from build123d import *

# Parameters (mm, degrees)
SKETCH2_W           = 42
SKETCH2_H           = 8.4
BOSS_EXTRUDE1_DEPTH = 2
SKETCH3_W           = 3.55
SKETCH3_H           = 8.4
SKETCH3_W_2         = 10
BOSS_EXTRUDE2_DEPTH = 2
FILLET1_R           = 2
SKETCH4_R           = 1
CUT_EXTRUDE1_DEPTH  = 2
SKETCH5_W           = 20
SKETCH5_H           = 28
BOSS_EXTRUDE3_DEPTH = 7.5
FILLET2_R           = 2
SKETCH6_W           = 3.5
SKETCH6_H           = 22
CUT_EXTRUDE2_DEPTH  = 20
SKETCH7_W           = 44.314231138
SKETCH7_H           = 10.974489351
CUT_EXTRUDE3_DEPTH  = 4
SKETCH8_W           = 14
SKETCH8_H           = 4
CUT_EXTRUDE4_DEPTH  = 10


with BuildPart() as part:
    # Sketch2 → Boss-Extrude1 (new body)
    with BuildSketch(Plane.XY.offset(-7.754792002)):
        Rectangle(SKETCH2_W, SKETCH2_H)
    extrude(amount=BOSS_EXTRUDE1_DEPTH)

    # Sketch3 → Boss-Extrude2 (add)
    with BuildSketch(Plane.XY.offset(-5.754792002)):
        with Locations((-8.975, 0)):
            Rectangle(SKETCH3_W, SKETCH3_H)
        with Locations((8.975, 0)):
            Rectangle(SKETCH3_W, SKETCH3_H)
        Rectangle(SKETCH3_W_2, SKETCH3_H)
    extrude(amount=BOSS_EXTRUDE2_DEPTH)

    # Fillet1
    fillet1_edges = [part.edges().sort_by_distance(p)[0] for p in [
        (-21, 4.2, -6.754792002),
        (21, 4.2, -6.754792002),
        (21, -4.2, -6.754792002),
        (-21, -4.2, -6.754792002),
    ]]
    fillet(fillet1_edges, radius=FILLET1_R)

    # Sketch4 → Cut-Extrude1 (cut)
    with BuildSketch(Plane.XY.offset(-5.754792002)):
        with Locations((-17.75, 0)):
            Circle(SKETCH4_R)
        with Locations((17.75, 0)):
            Circle(SKETCH4_R)
    extrude(amount=-CUT_EXTRUDE1_DEPTH, mode=Mode.SUBTRACT)

    # Sketch5 → Boss-Extrude3 (add)
    with BuildSketch(Plane(origin=(0, 0, -7.754792002), x_dir=(-1, 0, 0), z_dir=(0, 0, -1))):
        Rectangle(SKETCH5_W, SKETCH5_H)
    extrude(amount=BOSS_EXTRUDE3_DEPTH)

    # Fillet2
    fillet2_edges = [part.edges().sort_by_distance(p)[0] for p in [
        (0, 14, -7.754792002),
        (0, -14, -7.754792002),
        (0, 14, -15.254792002),
        (0, -14, -15.254792002),
    ]]
    fillet(fillet2_edges, radius=FILLET2_R)

    # Sketch6 → Cut-Extrude2 (cut)
    with BuildSketch(Plane.ZY.offset(10)):
        with Locations((-11.504792002, 0)):
            Rectangle(SKETCH6_W, SKETCH6_H)
    extrude(amount=-CUT_EXTRUDE2_DEPTH, mode=Mode.SUBTRACT)

    # Sketch7 → Cut-Extrude3 (cut)
    with BuildSketch(Plane.XY.offset(-3.754792002)):
        with Locations((-0.219821089, -0.04579799)):
            Rectangle(SKETCH7_W, SKETCH7_H)
    extrude(amount=-CUT_EXTRUDE3_DEPTH, mode=Mode.SUBTRACT)

    # Sketch8 → Cut-Extrude4 (cut)
    with BuildSketch(Plane.XY.offset(-7.754792002)):
        with Locations((0, -12)):
            Rectangle(SKETCH8_W, SKETCH8_H)
    extrude(amount=-CUT_EXTRUDE4_DEPTH, mode=Mode.SUBTRACT)


solid = part.part
Here's how the part is built. I have some questions about the finished solid (model axes, mm). A direction names the side the tool comes from. Give positions to 0.01 mm unless a question says otherwise; leave off trailing zeros. Write each loop counter-clockwise with the first axis right and the second up, starting at its lowest first coordinate (ties: lowest second). Pieces come first, ordered by that corner, then holes. Notation, with made-up numbers: (78.25, 50) -> (86.25, 50) arc R34 cw to (86.25, 85) -> close; hole circle Ø2 at (-33.5, 61.5). An arc over 180 degrees is marked (long way). Use one line per item in the form item = value. Start each with the question number.
1. Thinking about a two-plate mould opening in X: for faces 1 (the face through (10, 0, -9)), 2 (the face through (7, -12, -11)), 3 (the face through (0, 0, -9.755)), 4 (the face through (-7, -12, -11)), which applies, +X half, -X half, draft (parallel to the pull), parting line (faces both ways), or undercut?
2. Imagine slicing it at D-D on x = 9.25. List the corners of the cut face in (y, z) for me, plus the area to 3 significant figures.
3. Imagine slicing it at C-C on x = -2.5. List the corners of the cut face in (y, z) for me.
4. Imagine slicing it at B-B on y = -8.5. List the corners of the cut face in (x, z) for me.
5. Imagine slicing it at A-A on z = -12.5. List the corners of the cut face in (x, y) for me, plus the area to 3 significant figures.
6. If I drill on L1, parallel to Z at x = -2, y = 6.25; L2, parallel to Y at x = 8.75, z = -12.75; L3, parallel to X at y = -12.5, z = -12.75, over which ranges is the centre line in solid material (lowest first)?
7. On a 3-axis mill with a long thin cutter (end or side, diameter ignored), from which of +Z, -Z, +X, -X, +Y, -Y can I reach the whole of each face in a straight line? I mean faces 5 (the face through (9, -14, -11)), 6 (the face through (8, -11, -12)). Say none if no direction works.
8. Will these pins go through, and if not, where does the flat tip stop? pin 1 Ø8 at (x, y) = (-6.5, -11) entering from +Z; pin 2 Ø1 at (x, z) = (2, -14.5) entering from -Y.
Entries:
q1.face_1 = +X half
q1.face_2 = undercut
q1.face_3 = draft
q1.face_4 = undercut
q2.outline = (-14, -13.25) arc R2 ccw to (-12, -15.25) -> (12, -15.25) arc R2 ccw to (14, -13.25) -> (14, -9.75) arc R2 ccw to (12, -7.75) -> (-12, -7.75) arc R2 ccw to (-14, -9.75) -> close; hole (-11, -13.25) -> (11, -13.25) -> (11, -9.75) -> (-11, -9.75) -> close
q2.area = 130 mm²
q3.outline = (-10, -15.25) -> (12, -15.25) arc R2 ccw to (14, -13.25) -> (14, -9.75) arc R2 ccw to (12, -7.75) -> (-10, -7.75) -> (-10, -9.75) -> (11, -9.75) -> (11, -13.25) -> (-10, -13.25) -> close
q4.outline = (-10, -15.25) -> (10, -15.25) -> (10, -13.25) -> (-10, -13.25) -> close; (-10, -9.75) -> (10, -9.75) -> (10, -7.75) -> (-10, -7.75) -> close
q5.outline = (-10, -14) -> (-7, -14) -> (-7, -11) -> (-10, -11) -> close; (-10, 11) -> (10, 11) -> (10, 14) -> (-10, 14) -> close; (7, -14) -> (10, -14) -> (10, -11) -> (7, -11) -> close
q5.area = 78.0 mm²
q6.L1 = -15.25 to -13.25, -9.75 to -7.75
q6.L2 = -14 to -11, 11 to 14
q6.L3 = -10 to -7, 7 to 10
q7.face_5 = +Z, -Z, +X, -X, -Y
q7.face_6 = +X, -X
q8.pin_1 = -7.75
q8.pin_2 = -10
